Work out the finished part from the listing and answer in its coordinate system (mm). Coordinates: 2 decimals unless noted, no trailing zeros. Write each loop counter-clockwise with the first axis right and the second up, starting at its lowest first coordinate (ties: lowest second). Pieces come first, ordered by that corner, then holes. Notation, with made-up numbers: (-30, 81.25) - (26, 81.25) arc R31 cw to (26, 110.25) - close; hole circle Ø7 at (-39.5, -5). An arc over 180 degrees is marked (long way). Use a Markdown table: item, result. Add a question column.
(1) Given pin 1 Ø2.5 at (x, y) = (7.77, 66.5) entering from +Z; pin 2 Ø1 at (x, y) = (16.5, 32.5) entering from -Z (3 decimals), each flat-ended and moving along its own axis, determine where each tip first touches the part or whether it passes through.
(2) The part is cut by section B-B, the plane y = 120.3. Give the vertices of the cut face in (x, z) (3 decimals), then the cut area to 3 significant figures.
(3) The part is cut by section C-C, the plane y = 41.1. State how many separate pieces and enclosed holes the cut face has, then the cut area to 3 significant figures.
(4) The part is cut by section A-A, the plane z = -20.5. Give the vertices of the cut face in (x, y) (3 decimals).
(5) Find the intervals of material crossed by line 1 (Z direction, x = 23.5, y = 85.9); line 2 (X direction, y = 85.5, z = -16.25) (3 decimals); line 3 (Z direction, x = 16.75, y = 10.5) (3 decimals), in increasing order. Write a range as from..to.
(6) For a pull along Z with two mould halves and no side action, classify faces 1 (the face through (23.79, 117.751, -16.465)), 2 (the face through (8.574, 42.365, -1.565)), 3 (the face through (1.565, 92.351, -16.465)), 4 (the face through (2, 63, -25.4)) as released by +Z, released by -Z, zero draft, split by the parting line, or undercut.
from build123d import *

# Parameters (mm, degrees)
BOSS_EXTRUDE1_DEPTH = 127
SKETCH3_R           = 1.5
CUT_EXTRUDE1_DEPTH  = 132.982271537
SKETCH4_R           = 1.5
CUT_EXTRUDE2_DEPTH  = 10


with BuildPart() as part:
    # Sketch2 → Boss-Extrude1 (new body)
    with BuildSketch(Plane(origin=(0, 0, 0), x_dir=(1, 0, 0), z_dir=(0, 1, 0))):
        Polygon((22.225, 3.175), (12.7, 3.175), (3.175, 3.175), (3.175, 25.4), (0, 25.4), (0, 0), (25.4, 0), (25.4, 25.4), (22.225, 25.4), align=None)
    extrude(amount=BOSS_EXTRUDE1_DEPTH)

    # Sketch3 → Cut-Extrude1 (cut, through all)
    with BuildSketch(Plane.ZY):
        with Locations((-17.896152423, 9.7)):
            Circle(SKETCH3_R)
        with Locations((-17.896152423, 15.7)):
            Circle(SKETCH3_R)
        with Locations((-12.7, 18.7)):
            Circle(SKETCH3_R)
        with Locations((-12.7, 12.7)):
            Circle(SKETCH3_R)
        with Locations((-12.7, 6.7)):
            Circle(SKETCH3_R)
        with Locations((-7.503847577, 9.7)):
            Circle(SKETCH3_R)
        with Locations((-7.503847577, 15.7)):
            Circle(SKETCH3_R)
        with Locations((-17.896152423, 35.1)):
            Circle(SKETCH3_R)
        with Locations((-17.896152423, 41.1)):
            Circle(SKETCH3_R)
        with Locations((-12.7, 44.1)):
            Circle(SKETCH3_R)
        with Locations((-12.7, 38.1)):
            Circle(SKETCH3_R)
        with Locations((-7.503847577, 35.1)):
            Circle(SKETCH3_R)
        with Locations((-7.503847577, 41.1)):
            Circle(SKETCH3_R)
        with Locations((-12.7, 57.5)):
            Circle(SKETCH3_R)
        with Locations((-12.7, 63.5)):
            Circle(SKETCH3_R)
        with Locations((-12.7, 32.1)):
            Circle(SKETCH3_R)
        with Locations((-17.896152423, 60.5)):
            Circle(SKETCH3_R)
        with Locations((-17.896152423, 66.5)):
            Circle(SKETCH3_R)
        with Locations((-12.7, 69.5)):
            Circle(SKETCH3_R)
        with Locations((-7.503847577, 66.5)):
            Circle(SKETCH3_R)
        with Locations((-7.503847577, 60.5)):
            Circle(SKETCH3_R)
        with Locations((-17.896152423, 85.9)):
            Circle(SKETCH3_R)
        with Locations((-17.896152423, 91.9)):
            Circle(SKETCH3_R)
        with Locations((-12.7, 82.9)):
            Circle(SKETCH3_R)
        with Locations((-12.7, 88.9)):
            Circle(SKETCH3_R)
        with Locations((-7.503847577, 85.9)):
            Circle(SKETCH3_R)
        with Locations((-7.503847577, 91.9)):
            Circle(SKETCH3_R)
        with Locations((-12.7, 94.9)):
            Circle(SKETCH3_R)
        with Locations((-17.896152423, 111.3)):
            Circle(SKETCH3_R)
        with Locations((-12.7, 108.3)):
            Circle(SKETCH3_R)
        with Locations((-17.896152423, 117.3)):
            Circle(SKETCH3_R)
        with Locations((-12.7, 120.3)):
            Circle(SKETCH3_R)
        with Locations((-12.7, 114.3)):
            Circle(SKETCH3_R)
        with Locations((-7.503847577, 111.3)):
            Circle(SKETCH3_R)
        with Locations((-7.503847577, 117.3)):
            Circle(SKETCH3_R)
    extrude(amount=-CUT_EXTRUDE1_DEPTH, mode=Mode.SUBTRACT)

    # Sketch4 → Cut-Extrude2 (cut)
    with BuildSketch(Plane.XY):
        with BuildLine():
            Line((12.963682416, 112.8), (12.963682416, 114.3))
            Line((12.963682416, 114.3), (11.463682416, 114.3))
            ThreePointArc((11.463682416, 114.3), (11.903022244, 113.239339828), (12.963682416, 112.8))
        make_face()
        with Locations((12.963682416, 108.3)):
            Circle(SKETCH4_R)
        with Locations((7.767529993, 111.3)):
            Circle(SKETCH4_R)
        with Locations((7.767529993, 117.3)):
            Circle(SKETCH4_R)
        with Locations((12.963682416, 120.3)):
            Circle(SKETCH4_R)
        with Locations((18.159834839, 117.3)):
            Circle(SKETCH4_R)
        with Locations((18.159834839, 111.3)):
            Circle(SKETCH4_R)
        with Locations((12.963682416, 82.9)):
            Circle(SKETCH4_R)
        with Locations((12.963682416, 88.9)):
            Circle(SKETCH4_R)
        with Locations((12.963682416, 94.9)):
            Circle(SKETCH4_R)
        with Locations((18.159834839, 91.9)):
            Circle(SKETCH4_R)
        with Locations((18.159834839, 85.9)):
            Circle(SKETCH4_R)
        with Locations((7.767529993, 91.9)):
            Circle(SKETCH4_R)
        with Locations((7.767529993, 85.9)):
            Circle(SKETCH4_R)
        with Locations((12.963682416, 57.5)):
            Circle(SKETCH4_R)
        with Locations((12.963682416, 63.5)):
            Circle(SKETCH4_R)
        with Locations((12.963682416, 69.5)):
            Circle(SKETCH4_R)
        with Locations((18.159834839, 66.5)):
            Circle(SKETCH4_R)
        with Locations((18.159834839, 60.5)):
            Circle(SKETCH4_R)
        with Locations((7.767529993, 66.5)):
            Circle(SKETCH4_R)
        with Locations((7.767529993, 60.5)):
            Circle(SKETCH4_R)
        with Locations((12.963682416, 32.1)):
            Circle(SKETCH4_R)
        with Locations((12.963682416, 38.1)):
            Circle(SKETCH4_R)
        with Locations((12.963682416, 44.1)):
            Circle(SKETCH4_R)
        with Locations((18.159834839, 41.1)):
            Circle(SKETCH4_R)
        with Locations((18.159834839, 35.1)):
            Circle(SKETCH4_R)
        with Locations((7.767529993, 41.1)):
            Circle(SKETCH4_R)
        with Locations((7.767529993, 35.1)):
            Circle(SKETCH4_R)
        with Locations((12.963682416, 6.7)):
            Circle(SKETCH4_R)
        with Locations((12.963682416, 12.7)):
            Circle(SKETCH4_R)
        with Locations((12.963682416, 18.7)):
            Circle(SKETCH4_R)
        with Locations((18.159834839, 15.7)):
            Circle(SKETCH4_R)
        with Locations((18.159834839, 9.7)):
            Circle(SKETCH4_R)
        with Locations((7.767529993, 15.7)):
            Circle(SKETCH4_R)
        with Locations((7.767529993, 9.7)):
            Circle(SKETCH4_R)
    extrude(amount=-CUT_EXTRUDE2_DEPTH, mode=Mode.SUBTRACT)


solid = part.part
Model answer:
| question | item | result |
|---|---|---|
| 1 | pin 1 | through |
| 1 | pin 2 | z = -3.175 |
| 2 | outline | (0, -25.4) - (3.175, -25.4) - (3.175, -14.2) - (0, -14.2) - close; (0, -11.2) - (3.175, -11.2) - (3.175, -3.175) - (11.464, -3.175) - (11.464, 0) - (0, 0) - close; (14.464, -3.175) - (22.225, -3.175) - (22.225, -11.2) - (25.4, -11.2) - (25.4, 0) - (14.464, 0) - close; (22.225, -25.4) - (25.4, -25.4) - (25.4, -14.2) - (22.225, -14.2) - close |
| 2 | area | 193 mm^2 |
| 3 | separate pieces | 7 |
| 3 | enclosed holes | 0 |
| 3 | area | 165 mm^2 |
| 4 | outline | (0, 0) - (3.175, 0) - (3.175, 127) - (0, 127) - close; (22.225, 0) - (25.4, 0) - (25.4, 127) - (22.225, 127) - close |
| 5 | line 1 | -25.4..-19.4, -16.4..-9, -6..0 |
| 5 | line 2 | 0..3.175, 22.225..25.4 |
| 5 | line 3 | -3.175..0 |
| 6 | face 1 | undercut |
| 6 | face 2 | zero draft |
| 6 | face 3 | undercut |
| 6 | face 4 | released by -Z |
